Check sheet for the modelled part. Datum: model origin and axes. Units: mm. Round coordinates to 2 decimals unless told otherwise and drop trailing zeros. Order: outer loops, then holes, each group sorted by start corner. A loop starts at its lowest first (then second) coordinate and runs counter-clockwise, first axis right, second up.
```python
from build123d import *

# Parameters (mm, degrees)
SKETCH_1_R           = 50
SKETCH_1_R_2         = 40
EXTRUDE_1_DEPTH      = 50
EXTRUDE_2_REACH      = 238.327
EXTRUDE_2_END_RADIUS = 50
SKETCH_2_R           = 30


with BuildPart() as part:
    # 草图1 → 凸台-拉伸1 (new, symmetric)
    with BuildSketch(Plane(origin=(0, 0, 0), x_dir=(0, 0, -1), z_dir=(1, 0, 0))):
        Circle(SKETCH_1_R)
        Circle(SKETCH_1_R_2, mode=Mode.SUBTRACT)
    extrude_1 = extrude(amount=EXTRUDE_1_DEPTH, both=True)

    # 凸台-拉伸2: up to this cylinder (the profile starts outside it)
    extrude_2_end = Plane(origin=(0, 0, 0), z_dir=(-1, 0, 0)) * Cylinder(EXTRUDE_2_END_RADIUS, 577.654, mode=Mode.PRIVATE)
    # 草图2 → 凸台-拉伸2 (add, up to the surface)
    with BuildSketch(Plane(origin=(0, 175.5, 0), x_dir=(1, 0, 0), z_dir=(0, 1, 0)), mode=Mode.PRIVATE) as extrude_2_sk1:
        with Locations(Location((0, 0, 0), (0, 0, 270))):
            Circle(SKETCH_2_R)
    extrude_2_tool1 = extrude(extrude_2_sk1.sketch, amount=-EXTRUDE_2_REACH, mode=Mode.PRIVATE) - extrude_2_end
    extrude_2 = extrude_2_tool1.solids().sort_by_distance((0, 175.5, 0))[0]
    add(extrude_2)

    # 镜向2: 凸台-拉伸1, 凸台-拉伸2 across plane
    add(extrude_1.mirror(Plane.ZX.offset(175.5)))
    add(extrude_2.mirror(Plane.ZX.offset(175.5)))


solid = part.part
```
Item 1: Sectioned sample at C-C (x = 34.5). Record the cut outline in (y, z), and give its area (3 significant figures).
Answer:
outline: circle Ø100 at (0, 0); circle Ø100 at (351, 0); hole circle Ø80 at (0, 0); hole circle Ø80 at (351, 0)
area: 5,650 mm2
Item 2: Sectioned sample at D-D (x = 0). Record the cut outline in (y, z), and give its area (3 significant figures).
Answer:
outline: (40, -30) - (311, -30) arc R50 ccw (long way) to (311, 30) - (40, 30) arc R50 ccw (long way) to start; hole circle Ø80 at (0, 0); hole circle Ø80 at (351, 0)
area: 21,100 mm2
Item 3: Release check for a two-part mould opening along Y. For faces 1 (the cylindrical face through (1.32, 173.6, -29.97)), 2 (the flat face through (50, 317, 22)) record: released by +Y, released by -Y, zero draft, split by the parting line, or undercut.
Answer:
face 1: undercut
face 2: zero draft
Item 4: Sectioned sample at A-A (y = 0). Record the cut outline in (x, z).
Answer:
outline: (-50, -50) - (50, -50) - (50, -40) - (-50, -40) - close; (-50, 40) - (50, 40) - (50, 50) - (-50, 50) - close
Item 5: Sectioned sample at B-B (z = 0). Record the cut outline in (x, y).
Answer:
outline: (-50, -50) - (50, -50) - (50, -40) - (-50, -40) - close; (-50, 40) - (50, 40) - (50, 50) - (30, 50) - (30, 301) - (50, 301) - (50, 311) - (-50, 311) - (-50, 301) - (-30, 301) - (-30, 50) - (-50, 50) - close; (-50, 391) - (50, 391) - (50, 401) - (-50, 401) - close
Item 6: Scan lines: line 1 along Y through (x, z) = (25, 0); line 2 along Y through (x, z) = (-2, -31.5); line 3 along Y through (x, z) = (18.5, 10). Record each from-to range of solid material in increasing order.
Answer:
line 1: y = -50 to -40, 40 to 311, 391 to 401
line 2: y = -38.83 to -24.65, 24.65 to 38.83, 312.17 to 326.35, 375.65 to 389.83
line 3: y = -48.99 to -38.73, 38.73 to 312.27, 389.73 to 399.99
Item 7: Go/stop test with flat-tipped pins: P1, Ø8, axis at x = -18.5, z = -14.5, coming from the -Y side; P2, Ø3, axis at x = 33, z = -2, coming from the -Y side; P3, Ø2, axis at y = 77.5, z = -26, coming from the +X side; P4, Ø10, axis at y = 354, z = -37.5, coming from the +X side. Record where each tip stops, or that it passes through.
Answer:
P1: stops at y = -48.89
P2: stops at y = -50
P3: stops at x = 16.58
P4: stops at x = 50
